Can you work these out from the model? Positions are in its coordinate system, mm. A direction names the side the tool comes from. Round coordinates to 2 decimals unless told otherwise and drop trailing zeros. Order: outer loops, then holes, each group sorted by start corner. A loop starts at its lowest first (then second) coordinate and runs counter-clockwise, first axis right, second up. Notation, with made-up numbers: (80.5, -35.5) -> (90.5, -35.5) arc R16 ccw to (90.5, -27.5) -> close; hole circle Ø5 at (67, 25). An arc over 180 degrees is marked (long way). One line per item, written item: value.
```python
from build123d import *

# Parameters (mm, degrees)
SKETCH1_W                          = 12.8
SKETCH1_H                          = 15.5
BOSS_EXTRUDE1_DEPTH                = 21
SKETCH2_R                          = 5.5
SKETCH2_R_2                        = 3.2
BOSS_EXTRUDE2_DEPTH                = 9
SKETCH3_R                          = 4.075
BOSS_EXTRUDE3_DEPTH                = 3
BOSS_EXTRUDE3_TAPER                = 20
SKETCH6_W                          = 4.5
SKETCH6_H                          = 6.25
CUT_EXTRUDE1_DEPTH                 = 15.5
SKETCH7_W                          = 4.5
SKETCH7_H                          = 0.9
CUT_EXTRUDE2_DEPTH                 = 9
LPATTERN1_COUNT                    = 3
LPATTERN1_PITCH                    = 6.3
EXTRUDE_THIN1_DEPTH                = 2.25
SKETCH9_W                          = 3
SKETCH9_H                          = 0.5
EXTRUDE_THIN2_DEPTH                = 0.725
CHAMFER1_SIZE                      = 0.5
CHAMFER1_SIZE2                     = 0.866025404
CHAMFER1_PART_2_SIZE               = 0.5
CHAMFER1_PART_2_SIZE2              = 0.866025404
LPATTERN2_COUNT                    = 3
LPATTERN2_PITCH                    = 6.3
CHAMFER1_OF_LPATTERN2_SIZE2        = 0.5
CHAMFER1_OF_LPATTERN2_SIZE         = 0.866025404
CHAMFER1_PART_2_OF_LPATTERN2_SIZE2 = 0.5
CHAMFER1_PART_2_OF_LPATTERN2_SIZE  = 0.866025404


with BuildPart() as part:
    # Sketch1 → Boss-Extrude1 (new body)
    with BuildSketch(Plane(origin=(0, 0, 0), x_dir=(0, 0, -1), z_dir=(1, 0, 0))):
        with Locations((6.4, 7.75)):
            Rectangle(SKETCH1_W, SKETCH1_H)
    extrude(amount=BOSS_EXTRUDE1_DEPTH)

    # Sketch2 → Boss-Extrude2 (add)
    with BuildSketch(Plane.ZY):
        with Locations((-6.4, 9.05)):
            Circle(SKETCH2_R)
        with Locations((-6.4, 9.05)):
            Circle(SKETCH2_R_2, mode=Mode.SUBTRACT)
    extrude(amount=BOSS_EXTRUDE2_DEPTH)

    # Sketch3 → Boss-Extrude3 (add)
    with BuildSketch(Plane(origin=(21, 0, 0), x_dir=(0, 0, -1), z_dir=(1, 0, 0))):
        with Locations((6.4, 9.05)):
            Circle(SKETCH3_R)
    extrude(amount=BOSS_EXTRUDE3_DEPTH, taper=BOSS_EXTRUDE3_TAPER)

    # Sketch6 → Cut-Extrude1 (cut)
    with BuildSketch(Plane.XZ):
        with Locations((4.2, -3.125)):
            Rectangle(SKETCH6_W, SKETCH6_H)
    cut_extrude1 = extrude(amount=-CUT_EXTRUDE1_DEPTH, mode=Mode.SUBTRACT)

    # Sketch7 → Cut-Extrude2 (cut)
    with BuildSketch(Plane(origin=(0, 0, -12.8), x_dir=(-1, 0, 0), z_dir=(0, 0, -1))):
        with Locations((-4.2, 15.05)):
            Rectangle(SKETCH7_W, SKETCH7_H)
        with Locations((-4.2, 0.45)):
            Rectangle(SKETCH7_W, SKETCH7_H)
    cut_extrude2 = extrude(amount=-CUT_EXTRUDE2_DEPTH, mode=Mode.SUBTRACT)

    # LPattern1: Cut-Extrude1, Cut-Extrude2 ×3
    with Locations(*[(i * LPATTERN1_PITCH, 0, 0) for i in range(1, LPATTERN1_COUNT)]):
        add(cut_extrude1, mode=Mode.SUBTRACT)
        add(cut_extrude2, mode=Mode.SUBTRACT)

    # Sketch8 → Extrude-Thin1 (add, symmetric)
    with BuildSketch(Plane.ZY.offset(-4.2)):
        with BuildLine():
            Line((-6.25, 13.5), (-5.398229918, 13.5))
            ThreePointArc((-5.398229918, 13.5), (-5.084448593, 13.389283033), (-4.909630934, 13.106165118))
            Line((-4.909630934, 13.106165118), (-3.519996024, 6.710710403))
            Line((-3.519996024, 6.710710403), (-1.441008044, 2.470100604))
            ThreePointArc((-1.441008044, 2.470100604), (-1.465663914, 1.985472404), (-1.889957622, 1.75))
            Line((-1.889957622, 1.75), (-6.25, 1.75))
            Line((-6.25, 1.75), (-6.25, 1.25))
            Line((-6.25, 1.25), (-1.889957622, 1.25))
            ThreePointArc((-1.889957622, 1.25), (-1.041370205, 1.720944808), (-0.992058465, 2.690201208))
            Line((-0.992058465, 2.690201208), (-3.044298744, 6.876252459))
            Line((-3.044298744, 6.876252459), (-4.421031949, 13.212330236))
            ThreePointArc((-4.421031949, 13.212330236), (-4.770667267, 13.778566065), (-5.398229918, 14))
            Line((-5.398229918, 14), (-6.25, 14))
            Line((-6.25, 14), (-6.25, 13.5))
        make_face()
    extrude_thin1 = extrude(amount=EXTRUDE_THIN1_DEPTH, both=True)

    # Sketch9 → Extrude-Thin2 (add, symmetric)
    with BuildSketch(Plane.ZY.offset(-4.2)):
        with Locations((-14.3, 13.4)):
            Rectangle(SKETCH9_W, SKETCH9_H)
        with Locations((-14.3, 2.1)):
            Rectangle(SKETCH9_W, SKETCH9_H)
    extrude_thin2 = extrude(amount=EXTRUDE_THIN2_DEPTH, both=True)

    # Chamfer1
    chamfer1_edges = [part.edges().sort_by_distance(p)[0] for p in [
        (3.475, 13.4, -15.8),
        (4.925, 13.4, -15.8),
    ]]
    chamfer1_side = [part.faces().sort_by_distance(p)[0] for p in [
        (4.2, 13.4, -15.8),
    ]]
    chamfer(chamfer1_edges, length=CHAMFER1_SIZE, length2=CHAMFER1_SIZE2, reference=chamfer1_side[0])

    # Chamfer1 part 2
    chamfer1_part_2_edges = [part.edges().sort_by_distance(p)[0] for p in [
        (3.475, 2.1, -15.8),
        (4.925, 2.1, -15.8),
    ]]
    chamfer1_part_2_side = [part.faces().sort_by_distance(p)[0] for p in [
        (4.2, 2.1, -15.8),
    ]]
    chamfer(chamfer1_part_2_edges, length=CHAMFER1_PART_2_SIZE, length2=CHAMFER1_PART_2_SIZE2, reference=chamfer1_part_2_side[0])

    # LPattern2: Extrude-Thin1, Extrude-Thin2 ×3
    with Locations(*[(i * LPATTERN2_PITCH, 0, 0) for i in range(1, LPATTERN2_COUNT)]):
        add(extrude_thin1)
        add(extrude_thin2)

    # Chamfer1 of LPattern2
    chamfer1_of_lpattern2_edges = [part.edges().sort_by_distance(p)[0] for p in [
        (9.775, 13.4, -15.8),
        (11.225, 13.4, -15.8),
        (16.075, 13.4, -15.8),
        (17.525, 13.4, -15.8),
    ]]
    chamfer(chamfer1_of_lpattern2_edges, length=CHAMFER1_OF_LPATTERN2_SIZE, length2=CHAMFER1_OF_LPATTERN2_SIZE2)

    # Chamfer1 part 2 of LPattern2
    chamfer1_part_2_of_lpattern2_edges = [part.edges().sort_by_distance(p)[0] for p in [
        (9.775, 2.1, -15.8),
        (11.225, 2.1, -15.8),
        (16.075, 2.1, -15.8),
        (17.525, 2.1, -15.8),
    ]]
    chamfer(chamfer1_part_2_of_lpattern2_edges, length=CHAMFER1_PART_2_OF_LPATTERN2_SIZE, length2=CHAMFER1_PART_2_OF_LPATTERN2_SIZE2)


solid = part.part
```
Q1. Will these pins go through, and if not, where does the flat tip stop? pin 1 Ø0.6 at (y, z) = (2, -14) entering from +X (3 decimals); pin 2 Ø2 at (x, z) = (9.5, -8) entering from +Y; pin 3 Ø5 at (x, z) = (10.5, -4.5) entering from +Y; pin 4 Ø6 at (x, y) = (-4, 2) entering from +Z.
Answers below:
pin 1: x = 17.525
pin 2: y = 14.6
pin 3: y = 15.5
pin 4: z = -2.68
Q2. Please list where these lines run through material, in increasing order: line 1 along X through (y, z) = (5.25, -4); line 2 along X through (y, z) = (13, -1.5); line 3 along Y through (x, z) = (17.5, -5.75).
Answers below:
line 1: -9 to 1.95, 6.45 to 8.25, 12.75 to 14.55, 19.05 to 21
line 2: 0 to 1.95, 6.45 to 8.25, 12.75 to 14.55, 19.05 to 21
line 3: 1.25 to 1.75, 13.5 to 14
Q3. I want a section at B-B on x = -7. List the corners of the cut face in (y, z) for me, plus the area to 3 significant figures.
Answers below:
outline: circle Ø11 at (9.05, -6.4); hole circle Ø6.4 at (9.05, -6.4)
area: 62.9 mm^2
Q4. We'd pull the mould along Y, two halves only. Please class faces 1 (the face through (10.468, 4.62, -2.495)), 2 (the face through (8.25, 8, -3)), 3 (the face through (10.468, 10, -3.723)), 4 (the face through (6.45, 6, -4)): released by +Y, released by -Y, zero draft, split by the parting line, or undercut.
Answers below:
face 1: undercut
face 2: zero draft
face 3: released by +Y
face 4: undercut
Q5. I want a section at A-A on z = -14.25. List the corners of the cut face in (x, y) for me (3 decimals).
Answers below:
outline: (3.475, 1.85) -> (4.925, 1.85) -> (4.925, 2.35) -> (3.475, 2.35) -> close; (3.475, 13.15) -> (4.925, 13.15) -> (4.925, 13.65) -> (3.475, 13.65) -> close; (9.775, 1.85) -> (11.225, 1.85) -> (11.225, 2.35) -> (9.775, 2.35) -> close; (9.775, 13.15) -> (11.225, 13.15) -> (11.225, 13.65) -> (9.775, 13.65) -> close; (16.075, 1.85) -> (17.525, 1.85) -> (17.525, 2.35) -> (16.075, 2.35) -> close; (16.075, 13.15) -> (17.525, 13.15) -> (17.525, 13.65) -> (16.075, 13.65) -> close
Q6. I want a section at C-C on y = 9.05. Give the number of separate pieces and of enclosed holes in the cut face, plus the area to 3 significant figures.
Answers below:
separate pieces: 1
enclosed holes: 3
area: 254 mm^2
Q7. On a 3-axis mill with a long thin cutter (end or side, diameter ignored), from which of +Z, -Z, +X, -X, +Y, -Y can I reach the whole of each face in a straight line? I mean faces 5 (the face through (4, 1.75, -4)), 6 (the face through (4.2, 13.8, -4.8)), 7 (the face through (-4.44, 11.21, -8.76)). Say none if no direction works.
Answers below:
face 5: none
face 6: +Z, +Y
face 7: -X
